Model file for the job. Use its own axes, mm. A direction names the side the tool comes from. Coordinates: 2 decimals unless noted, no trailing zeros. Write each loop counter-clockwise with the first axis right and the second up, starting at its lowest first coordinate (ties: lowest second). Pieces come first, ordered by that corner, then holes. Notation, with made-up numbers: (31, 17.5) -> (43, 17.5) arc R24 ccw to (43, 31.5) -> close; hole circle Ø3 at (81, -32.5). An arc over 180 degrees is marked (long way). Write item = value, one per line. Start each with the question number.
from build123d import *

# Parameters (mm, degrees)
SKETCH1_W           = 200
SKETCH1_H           = 150
BOSS_EXTRUDE1_DEPTH = 6
SKETCH3_W           = 100
SKETCH3_H           = 97.5
CUT_EXTRUDE1_DEPTH  = 6
BOSS_EXTRUDE3_DEPTH = 6
SKETCH5_W           = 6
SKETCH5_H           = 15
CUT_EXTRUDE2_DEPTH  = 6
SKETCH6_W           = 6
SKETCH6_H           = 37.5
CUT_EXTRUDE3_DEPTH  = 6
SKETCH8_W           = 350
SKETCH8_H           = 100
BOSS_EXTRUDE4_DEPTH = 6
LPATTERN1_COUNT     = 3
LPATTERN1_PITCH     = 75
SKETCH7_W           = 15
SKETCH7_H           = 6
CUT_EXTRUDE_S_DEPTH = 381.835922675


with BuildPart() as part:
    # Sketch1 → Boss-Extrude1 (new body)
    with BuildSketch(Plane.XY):
        with Locations((-100, 75)):
            Rectangle(SKETCH1_W, SKETCH1_H)
        with BuildLine():
            Line((-175, 110), (-175, 125))
            Line((-175, 125), (-25, 125))
            Line((-25, 125), (-25, 110))
            ThreePointArc((-25, 110), (-30.691670032, 81.340701386), (-46.902810588, 57.03125))
            ThreePointArc((-46.902810588, 57.03125), (-100, 27.5), (-153.097189412, 57.03125))
            ThreePointArc((-153.097189412, 57.03125), (-169.308329968, 81.340701386), (-175, 110))
        make_face(mode=Mode.SUBTRACT)
    extrude(amount=BOSS_EXTRUDE1_DEPTH)

    # Sketch3 → Cut-Extrude1 (cut)
    with BuildSketch(Plane.XY.offset(6)):
        with Locations((-150, 76.25)):
            Rectangle(SKETCH3_W, SKETCH3_H)
    extrude(amount=-CUT_EXTRUDE1_DEPTH, mode=Mode.SUBTRACT)

    # Sketch4 → Boss-Extrude3 (add)
    with BuildSketch(Plane.XY.offset(6)):
        with BuildLine():
            Line((-200, 27.5), (-250, 27.5))
            ThreePointArc((-250, 27.5), (-280.378472024, 35.379505335), (-303.097189412, 57.03125))
            ThreePointArc((-303.097189412, 57.03125), (-319.308329968, 81.340701386), (-325, 110))
            Line((-325, 110), (-325, 125))
            Line((-325, 125), (-200, 125))
            Line((-200, 125), (-200, 150))
            Line((-200, 150), (-350, 150))
            Line((-350, 150), (-350, 0))
            Line((-350, 0), (-200, 0))
            Line((-200, 0), (-200, 27.5))
        make_face()
    extrude(amount=-BOSS_EXTRUDE3_DEPTH)

    # Sketch5 → Cut-Extrude2 (cut)
    with BuildSketch(Plane.XY.offset(6)):
        with Locations((-175, 142.5)):
            Rectangle(SKETCH5_W, SKETCH5_H)
        with Locations((-175, 20)):
            Rectangle(SKETCH5_W, SKETCH5_H)
    extrude(amount=-CUT_EXTRUDE2_DEPTH, mode=Mode.SUBTRACT)

    # Sketch6 → Cut-Extrude3 (cut)
    with BuildSketch(Plane.XY.offset(6)):
        with Locations((-3, 93.75)):
            Rectangle(SKETCH6_W, SKETCH6_H)
    cut_extrude3 = extrude(amount=-CUT_EXTRUDE3_DEPTH, mode=Mode.SUBTRACT)

    # Sketch8 → Boss-Extrude4 (add)
    with BuildSketch(Plane.XY.offset(6)):
        with Locations((-175, -50)):
            Rectangle(SKETCH8_W, SKETCH8_H)
    extrude(amount=-BOSS_EXTRUDE4_DEPTH)

    # LPattern1: Cut-Extrude3 ×3
    with Locations(*[(0, -i * LPATTERN1_PITCH, 0) for i in range(1, LPATTERN1_COUNT)]):
        add(cut_extrude3, mode=Mode.SUBTRACT)

    # Sketch7 → Cut-Extrude s (cut, through all)
    with BuildSketch(Plane.XY.offset(6)):
        with Locations((-23.5, -97)):
            Rectangle(SKETCH7_W, SKETCH7_H)
        with Locations((-195.5, -97)):
            Rectangle(SKETCH7_W, SKETCH7_H)
    extrude(amount=-CUT_EXTRUDE_S_DEPTH, mode=Mode.SUBTRACT)


solid = part.part
(1) Drop flat-ended pins along their axis: pin 1 Ø1.8 at (x, z) = (-194, 1.5) entering from -Y; pin 2 Ø3 at (y, z) = (92.5, 1.5) entering from +X. Give the stop position or say it passes through.
(2) Saw through at B-B (y = 47). Give the cut face in (x, z).
(3) Mould opens along Y. For faces 1 (the face through (-279.99, 35.165, 3.042)), 2 (the face through (-177, -1, 0)) say: released by +Y, released by -Y, zero draft, split by the parting line, or undercut.
(4) 3-axis set-ups, long thin cutter, end or side, ignore diameter. For faces 3 (the face through (-30.535, 81.722, 2.958)), 4 (the face through (-177, -1, 6)): which of +Z, -Z, +X, -X, +Y, -Y reach the whole face in a straight line?
(5) Saw through at C-C (y = -42.5). Give the cut face in (x, z), then the cut area to 3 significant figures.
(6) Drill centre lines: line 1 along X through (y, z) = (26, 2.6); line 2 along Y through (x, z) = (-145.5, 0.75); line 3 along X through (y, z) = (117, 4.4). Where is each one in solid material? Low to high.
(7) Saw through at A-A (x = -243). Give the cut face in (y, z).
Returned:
q1.pin_1 = -94
q1.pin_2 = -6
q2.outline = (-350, 0) -> (-295.36, 0) -> (-295.36, 6) -> (-350, 6) -> close; (-54.64, 0) -> (0, 0) -> (0, 6) -> (-54.64, 6) -> close
q3.face_1 = undercut
q3.face_2 = zero draft
q4.face_3 = +Z, -Z
q4.face_4 = +Z, +X, -X, +Y, -Y
q5.outline = (-350, 0) -> (-6, 0) -> (-6, 6) -> (-350, 6) -> close
q5.area = 2,060 mm2
q6.line_1 = -350 to -178, -172 to -6
q6.line_2 = -100 to 27.5, 125 to 150
q6.line_3 = -350 to -325, -25 to 0
q7.outline = (-100, 0) -> (27.5, 0) -> (27.5, 6) -> (-100, 6) -> close; (125, 0) -> (150, 0) -> (150, 6) -> (125, 6) -> close
